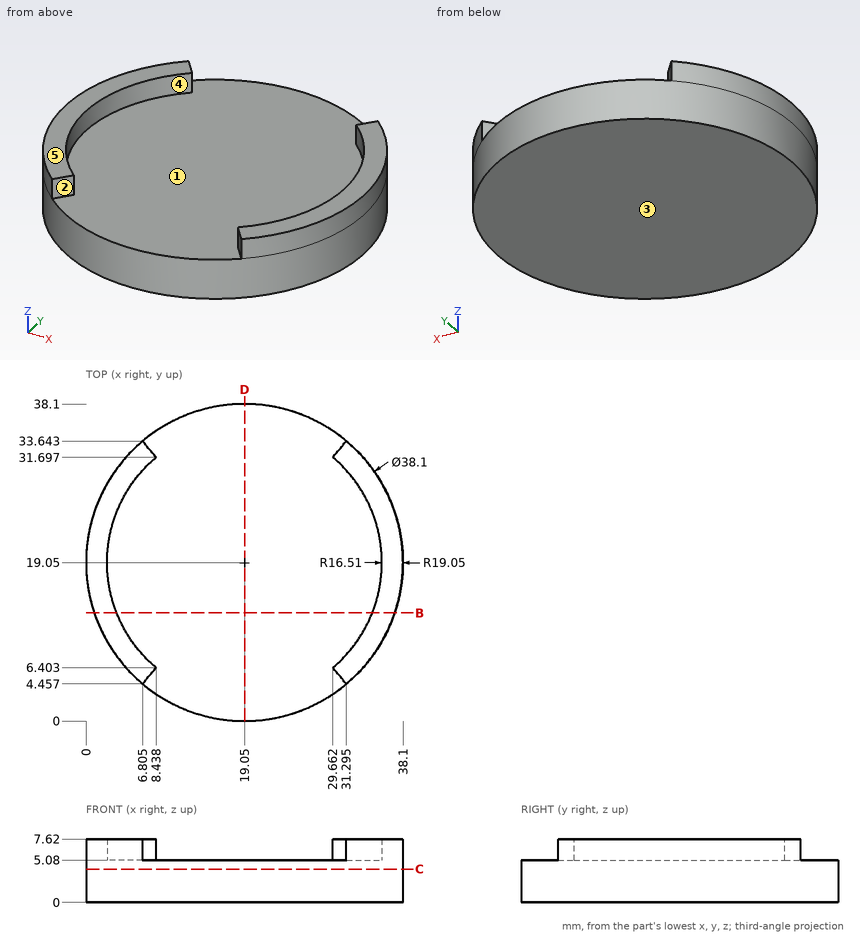
The figure shows three views and two pictorial views of one solid part (mm, origin at its lowest corner). Answer the questions. A direction names the side the tool comes from. Coordinates: 2 decimals unless noted, no trailing zeros. Write each loop counter-clockwise with the first axis right and the second up, starting at its lowest first coordinate (ties: lowest second). Pieces come first, ordered by that corner, then holes. Notation, with made-up numbers: (69, -19) -> (104, -19) arc R26 ccw to (104, 12) -> close; hole circle Ø10 at (41.5, 39). An arc over 180 degrees is marked (long way). Return JSON: item names as keys, results as strings.
(1) The part is cut by section D-D on x = 19.05. Give the vertices of the cut face in (y, z).
Answers below:
{"outline": "(0, 0) -> (38.1, 0) -> (38.1, 5.08) -> (0, 5.08) -> close"}
(2) The part is cut by section B-B on y = 13. Give the vertices of the cut face in (x, z), then the cut area to 3 significant figures.
Answers below:
{"outline": "(0.99, 0) -> (37.11, 0) -> (37.11, 7.62) -> (34.41, 7.62) -> (34.41, 5.08) -> (3.69, 5.08) -> (3.69, 7.62) -> (0.99, 7.62) -> close", "area": "197 mm^2"}
(3) Each of these flat-tipped pins is pushed along its axis until it touches: P1, Ø1.5, axis at y = 4.5, z = 5.5, coming from the -X side; P2, Ø5, axis at x = 21.5, y = 16.5, coming from the +Z side. Where does it stop, or does it pass through?
Answers below:
{"P1": "x = 5.92", "P2": "z = 5.08"}
(4) Consider line 1 along Z through (x, y) = (30.5, 30); line 2 along X through (y, z) = (27.5, 6.25) (1 decimal); line 3 along Y through (x, z) = (5.5, 1). Determine where each line is inside the solid, lowest interval first. Write a range as from..to.
Answers below:
{"line 1": "0..5.08", "line 2": "2..4.9, 33.2..36.1", "line 3": "5.66..32.44"}
(5) Which of the six approach directions +Z, -Z, +X, -X, +Y, -Y give full straight-line access (tool end or side, diameter ignored) to the marked faces 4 and 5?
Answers below:
{"face 4": "+Z", "face 5": "+Z, +X, -X, +Y, -Y"}
(6) For a pull along X with two mould halves and no side action, classify the marked faces 1, 2 and 3 as pulls with the +X half, pulls with the -X half, needs draft (parallel to the pull), parting line crosses it, or undercut.
Answers below:
{"face 1": "undercut", "face 2": "undercut", "face 3": "needs draft"}
(7) The part is cut by section C-C on z = 4. Give the vertices of the cut face in (x, y), then the cut area to 3 significant figures.
Answers below:
{"outline": "circle Ø38.1 at (19.05, 19.05)", "area": "1,140 mm^2"}
